Autodesk Inventor part; units mm, degrees
ref_plane "YZ Plane" through (0, 0, 0) normal (1, 0, 0) x (0, 1, 0)
ref_plane "XZ Plane" through (0, 0, 0) normal (0, 1, 0) x (-1, 0, 0)
ref_plane "XY Plane" through (0, 0, 0) normal (0, 0, 1) x (1, 0, 0)
sketch "Sketch1" plane through (0, 0, 0) normal (0, 1, 0) x (-1, 0, 0)
  line L0 (0, 0) -> (25.2, 0)
  line L1 (25.2, 0) -> (25.2, -32.2)
  line L2 (25.2, -32.2) -> (0, -32.2)
  line L3 (0, -32.2) -> (0, 0)
  line L4 (15.7, -11.2) -> (9.5, -11.2)
  line L5 (9.5, -11.2) -> (9.5, -21)
  line L6 (9.5, -21) -> (15.7, -21)
  line L7 (15.7, -21) -> (15.7, -11.2)
  circle A0 centre (20.6, -8.1) radius 1.25
  circle A1 centre (20.6, -16.1) radius 1.25
  circle A2 centre (20.6, -24.1) radius 1.25
  circle A3 centre (12.6, -8.1) radius 1.25
  circle A4 centre (12.6, -16.1) radius 1.25
  circle A5 centre (12.6, -24.1) radius 1.25
  circle A6 centre (4.6, -8.1) radius 1.25
  circle A7 centre (4.6, -16.1) radius 1.25
  circle A8 centre (4.6, -24.1) radius 1.25
  dimension "d0" = 25.2
  dimension "d1" = 32.2
  dimension "d2" = 9.5
  dimension "d3" = 9.5
  dimension "d4" = 11.2
  dimension "d5" = 11.2
  dimension "d6" = 2.5
  dimension "d9" = 8
  dimension "d12" = 8
  dimension "d15" = 4.6
  dimension "d16" = 4.6
  dimension "d17" = 16.1
  dimension "d18" = 16.1
extrude "Extrusion1" add sketch "Sketch1" along normal blind 4 contours L0 L1 L2 L3
sketch "Sketch2" plane through (-25.2, 0, 0) normal (0, 0, 1) x (1, 0, 0)
  line L0 (0, 0) -> (0, 4)
  line L1 (0, 4) -> (25.2, 4)
  line L2 (25.2, 4) -> (25.2, -5)
  line L3 (25.2, -5) -> (0, -5)
  line L4 (0, -5) -> (0, 4)
  circle A0 centre (4.6, -1) radius 1
  circle A1 centre (20.6, -1) radius 1
  point P0 (25.2, 0)
  dimension "d21" = 9
  dimension "d22" = 25.2
  dimension "d23" = 2
  dimension "d24" = 2
  dimension "d25" = 4.6
  dimension "d26" = 4.6
  dimension "d27" = 5
  dimension "d28" = 5
extrude "Extrusion2" add sketch "Sketch2" along normal blind 3
sketch "Sketch3" plane through (0, 0, -32.2) normal (0, 0, -1) x (-1, 0, 0)
  line L0 (0, 0) -> (0, 4)
  line L1 (0, 4) -> (25.2, 4)
  line L2 (25.2, 4) -> (25.2, -5)
  line L3 (25.2, -5) -> (0, -5)
  line L4 (0, -5) -> (0, 4)
  circle A0 centre (4.6, -1) radius 1
  circle A1 centre (20.6, -1) radius 1
  point P0 (25.2, 0)
  dimension "d31" = 9
  dimension "d32" = 25.2
  dimension "d33" = 2
  dimension "d34" = 2
  dimension "d35" = 4.6
  dimension "d36" = 4.6
  dimension "d37" = 5
  dimension "d38" = 5
extrude "Extrusion3" add sketch "Sketch3" along normal blind 3
chamfer "Chamfer1" distance 2 angle 45 6 edges at (-12.6, 4, -35.2) (-12.6, 4, 3) (0, -5, 1.5) (-25.2, -5, 1.5) (-25.2, -5, -33.7) (0, -5, -33.7)
equation "\"d3\" = d2"
equation "\"d5\" = d4"
equation "\"d15\" = d16"
equation "\"d17\" = d18"
equation "\"d24\" = d23"
equation "\"d26\" = d25"
equation "\"d28\" = d27"
equation "\"d34\" = d33"
equation "\"d36\" = d35"
equation "\"d38\" = d37"
properties part number "fixation_ax12" material "ABS Plastic"
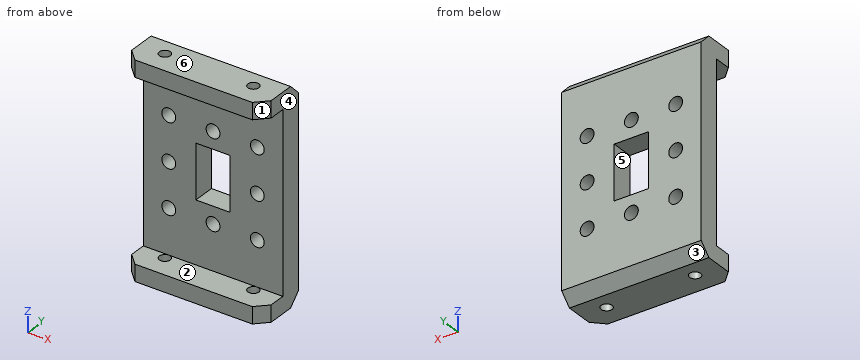
Can you work these out from the model? Positions are in its coordinate system, mm. Face numbers are marked on the shaded views. A direction names the side the tool comes from. Give positions to 0.01 mm unless a question says otherwise; leave off trailing zeros. Order: outer loops, then holes, each group sorted by start corner. A loop starts at its lowest first (then second) coordinate and runs counter-clockwise, first axis right, second up. Notation, with made-up numbers: M -0.75,86 L 5.25,86 A20 cw 5.25,108 Z; hole C 71.25,64.5 d11. An arc over 180 degrees is marked long. Use one line per item in the form item = value. Start each with the question number.
Item 1: If we section it at A-A (x = -10): Write out the boundary of the cut face in (y, z).
Item 2: Will these pins go through, and if not, where does the flat tip stop? pin 1 Ø1.5 at (x, z) = (-5, -8.5) entering from -Y; pin 2 Ø1.2 at (x, y) = (-4.6, -1) entering from -Z.
Item 3: For the marked faces 1 and 2, which set-ups out of +Z, -Z, +X, -X, +Y, -Y let a thin tool reach every point of the face, with its end or its side?
Item 4: If we section it at C-C (y = -4.25): Write out the boundary of the cut face in (x, z).
Item 5: If we section it at D-D (x = -12.6): Write out the boundary of the cut face in (y, z), then the cut area to 3 significant figures.
Item 6: If we section it at B-B (z = -24.1): Write out the boundary of the cut face in (x, y), then the cut area to 3 significant figures.
Item 7: We'd pull the mould along Z, two halves only. Please class the marked faces 3, 4, 5 and 6: +Z half, -Z half, draft (parallel to the pull), parting line (faces both ways), or undercut.
Item 8: If I drill on line 1 along X through (y, z) = (-1, 1.3); line 2 along Z through (x, y) = (-18.75, -1.75); line 3 along X through (y, z) = (1.5, -7.5), over which ranges is the centre line in solid material (lowest first)?
Outcome:
q1.outline = M -5,-35.2 L 2,-35.2 L 4,-33.2 L 4,-21 L 0,-21 L 0,-32.2 L -5,-32.2 Z; M -5,0 L 0,0 L 0,-11.2 L 4,-11.2 L 4,1 L 2,3 L -5,3 Z
q2.pin_1 = 0
q2.pin_2 = through
q3.face_1 = +Z, -Z, +X, -Y
q3.face_2 = +X, -X, -Y
q4.outline = M -23.95,-35.2 L -1.25,-35.2 L -1.25,-32.2 L -23.95,-32.2 Z; M -23.95,0 L -1.25,0 L -1.25,3 L -23.95,3 Z
q5.outline = M -5,-35.2 L 2,-35.2 L 4,-33.2 L 4,-25.35 L 0,-25.35 L 0,-32.2 L -5,-32.2 Z; M -5,0 L 0,0 L 0,-6.85 L 4,-6.85 L 4,1 L 2,3 L -5,3 Z; M 0,-22.85 L 4,-22.85 L 4,-21 L 0,-21 Z; M 0,-11.2 L 4,-11.2 L 4,-9.35 L 0,-9.35 Z
q5.area = 120 mm2
q6.outline = M -25.2,0 L -21.85,0 L -21.85,4 L -25.2,4 Z; M -19.35,0 L -13.85,0 L -13.85,4 L -19.35,4 Z; M -11.35,0 L -5.85,0 L -5.85,4 L -11.35,4 Z; M -3.35,0 L 0,0 L 0,4 L -3.35,4 Z
q6.area = 70.8 mm2
q7.face_3 = -Z half
q7.face_4 = draft
q7.face_5 = undercut
q7.face_6 = +Z half
q8.line_1 = -25.2 to -21.6, -19.6 to -5.6, -3.6 to 0
q8.line_2 = -35.2 to -32.2, 0 to 3
q8.line_3 = -25.2 to -21.7, -19.5 to -13.7, -11.5 to -5.7, -3.5 to 0
